Work out the finished part from the listing and answer in its coordinate system (mm). Round coordinates to 2 decimals unless told otherwise and drop trailing zeros. Order: outer loops, then holes, each group sorted by start corner. A loop starts at its lowest first (then second) coordinate and runs counter-clockwise, first axis right, second up. Notation, with made-up numbers: (-14.75, -3.75) - (27.25, -3.75) arc R27 ccw to (27.25, 33.25) - close; hole circle Ø2 at (57, -7.75). An arc over 180 degrees is marked (long way). Put each result on its own line as item: value.
Autodesk Inventor part; units mm, degrees
ref_plane "YZ Plane" through (0, 0, 0) normal (1, 0, 0) x (0, 1, 0)
ref_plane "XZ Plane" through (0, 0, 0) normal (0, 1, 0) x (-1, 0, 0)
ref_plane "XY Plane" through (0, 0, 0) normal (0, 0, 1) x (1, 0, 0)
sketch "Sketch3" plane through (-10.4876, -69.85, 2.286) normal (0, -1, 0) x (1, 0, 0)
  line L0 (0, 0) -> (22.7558, 0)
  line L1 (0, -2.286) -> (0, 0)
  line L2 (0, -2.286) -> (22.7558, -2.286)
  line L3 (22.7558, -2.286) -> (22.7558, 0)
  line L4 (22.7558, 0) -> (23.3146, 0)
  line L5 (22.7558, -2.286) -> (22.7558, 0)
  line L6 (22.7558, -2.286) -> (23.3146, -2.286)
  line L7 (23.3146, -2.286) -> (23.3146, 0)
  line L8 (0, 0) -> (-2.0854, 0)
  line L9 (-2.0854, -2.286) -> (-2.0854, 0)
  line L10 (0, -2.286) -> (-2.0854, -2.286)
  line L11 (0, -2.286) -> (0, 0)
  point P0 (10.4876, -2.286)
extrude "Extrusion3" add sketch "Sketch3" along normal mid plane 38.1
sketch "Sketch4" plane through (65.7357, -25.8425, 2.286) normal (0.866, -0.5, 0) x (0, 0, -1)
  line L0 (2.286, 0) -> (0, 0)
  line L1 (0, -22.7558) -> (0, 0)
  line L2 (2.286, -22.7558) -> (0, -22.7558)
  line L3 (2.286, -22.7558) -> (2.286, 0)
  line L4 (0, 0) -> (0, 2.0854)
  line L5 (2.286, 0) -> (0, 0)
  line L6 (2.286, 0) -> (2.286, 2.0854)
  line L7 (2.286, 2.0854) -> (0, 2.0854)
  line L8 (0, -23.3146) -> (0, -22.7558)
  line L9 (2.286, -23.3146) -> (0, -23.3146)
  line L10 (2.286, -23.3146) -> (2.286, -22.7558)
  line L11 (2.286, -22.7558) -> (0, -22.7558)
  point P0 (2.286, -10.4876)
extrude "Extrusion4" add sketch "Sketch4" along normal mid plane 38.1
sketch "Sketch5" plane through (12.827, -88.9, 0) normal (0, 0, -1) x (-1, 0, 0)
  arc A0 (-30.132, 61.7072) -> (-32.2021, 65.2928) centre (-31.1671, 63.5) ccw
  line L0 (-32.2021, 65.2928) -> (-30.132, 61.7072)
  line L1 (7.3756, 100.2707) -> (-70.4492, 55.3385)
  line L2 (-57.7492, 33.3415) -> (-70.4492, 55.3385)
  line L3 (-4.7625, 63.9334) -> (-57.7492, 33.3415)
  arc A1 (0, 61.1837) -> (-4.7625, 63.9334) centre (-3.175, 61.1837) ccw
  line L4 (0, 61.1837) -> (0, 0)
  line L5 (25.4, 0) -> (0, 0)
  line L6 (25.4, 89.8643) -> (25.4, 0)
  line L7 (24.8412, 91.9497) -> (25.4, 89.8643)
  line L8 (9.461, 100.8295) -> (24.8412, 91.9497)
  line L9 (9.461, 100.8295) -> (7.3756, 100.2707)
  arc A2 (14.8971, 38.1) -> (10.7569, 38.1) centre (12.827, 38.1) ccw
  line L10 (10.7569, 38.1) -> (14.8971, 38.1)
  circle A3 centre (-9.17, 76.2) radius 2.0701
  circle A4 centre (12.827, 88.9) radius 2.0701
  circle A5 centre (12.827, 63.5) radius 2.0701
extrude "Extrusion5" add sketch "Sketch5" against normal blind 2.286
sketch "Sketch6" plane through (12.827, -88.9, 0) normal (0, 0, -1) x (-1, 0, 0)
  arc A0 (-30.132, 61.7072) -> (-32.2021, 65.2928) centre (-31.1671, 63.5) ccw
  line L0 (-57.7492, 33.3415) -> (-70.4492, 55.3385)
  line L1 (-4.7625, 63.9334) -> (-57.7492, 33.3415)
  line L2 (25.4, 89.8643) -> (25.4, 0)
  arc A1 (14.8971, 38.1) -> (10.7569, 38.1) centre (12.827, 38.1) ccw
  circle A2 centre (-9.17, 76.2) radius 2.0701
  circle A3 centre (12.827, 88.9) radius 2.0701
  circle A4 centre (12.827, 63.5) radius 2.0701
  circle A5 centre (12.827, 88.9) radius 2.54
  circle A6 centre (-9.17, 76.2) radius 2.54
  circle A7 centre (12.827, 63.5) radius 2.54
  circle A8 centre (12.827, 38.1) radius 2.54
  circle A9 centre (-31.1671, 63.5) radius 2.54
  circle A10 centre (-53.1006, 50.69) radius 2.54
  circle A11 centre (12.7, 12.7) radius 2.54
  dimension "d20" = 5.08
  dimension "d21" = 5.08
  dimension "d22" = 5.08
  dimension "d23" = 5.08
  dimension "d24" = 5.08
  dimension "d25" = 5.08
  dimension "d26" = 5.08
  dimension "d27" = 12.7
  dimension "d28" = 25.4
  dimension "d29" = 12.7
  dimension "d30" = 12.7
extrude "Extrusion6" cut sketch "Sketch6" against normal blind 2.286 contours A2 | A3 | A4 | A5 | A6 | A7 | A8 | A9 | A10 | A11
sketch "Sketch7" plane through (12.827, -88.9, 0) normal (0, 0, -1) x (-1, 0, 0)
  circle A0 centre (12.827, 38.1) radius 2.54
  circle A1 centre (-31.1671, 63.5) radius 2.54
  line L0 (-4.7625, 63.9334) -> (-57.7492, 33.3415)
  arc A2 (0, 61.1837) -> (-4.7625, 63.9334) centre (-3.175, 61.1837) ccw
  line L1 (0, 61.1837) -> (0, 0)
  line L2 (-31.1671, 63.5) -> (12.827, 38.1) construction
  line L3 (-18.3401, 56.0943) -> (0, 66.683)
  line L4 (0, 66.683) -> (0, 45.5057)
  line L5 (0, 61.1837) -> (0, 0)
  line L6 (0, 45.5057) -> (-18.3401, 56.0943)
extrude "Extrusion7" add sketch "Sketch7" against normal blind 2.286 contours A2 L1 L6 L0
properties part number "Versaframe 60deg gusset" material "Aluminum 6061"
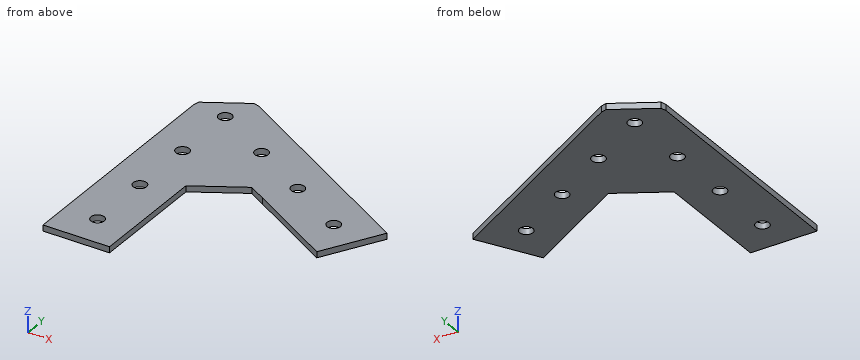
1) A cutting plane is placed at B-B on x = 0. Write down the section's boundary in (y, z), then the cut area to 3 significant figures.
Findings below:
outline: (-88.9, 0) - (-78.74, 0) - (-78.74, 2.29) - (-88.9, 2.29) - close; (-73.66, 0) - (-53.34, 0) - (-53.34, 2.29) - (-73.66, 2.29) - close; (-48.26, 0) - (-27.94, 0) - (-27.94, 2.29) - (-48.26, 2.29) - close; (-22.86, 0) - (-2.54, 0) - (-2.54, 2.29) - (-22.86, 2.29) - close; (2.54, 0) - (9.99, 0) - (9.99, 2.29) - (2.54, 2.29) - close
area: 180 mm2
2) Straight lines are drawn through the part: L1, parallel to Y at x = 0, z = 1.25; L2, parallel to X at y = -52, z = 0.95; L3, parallel to Y at x = 42.5, z = 0.6. For each, find the intervals that lie inside material, in ascending order. Write a range as from..to.
Findings below:
L1: y = -88.9..-78.74, -73.66..-53.34, -48.26..-27.94, -22.86..-2.54, 2.54..9.99
L2: x = -12.57..-2.24, 2.24..12.83, 64.41..72.63
L3: y = -39.35..-27.45, -23.35..-10.02
3) A cutting plane is placed at D-D on y = -12.7. Write down the section's boundary in (x, z).
Findings below:
outline: (-12.57, 0) - (19.46, 0) - (19.46, 2.29) - (-12.57, 2.29) - close; (24.54, 0) - (47.14, 0) - (47.14, 2.29) - (24.54, 2.29) - close
4) A cutting plane is placed at A-A on y = -25.4. Write down the section's boundary in (x, z).
Findings below:
outline: (-12.57, 0) - (-2.54, 0) - (-2.54, 2.29) - (-12.57, 2.29) - close; (2.54, 0) - (41.45, 0) - (41.45, 2.29) - (2.54, 2.29) - close; (46.53, 0) - (69.14, 0) - (69.14, 2.29) - (46.53, 2.29) - close
5) A cutting plane is placed at C-C on z = 1.25. Give the number of separate pieces and of enclosed holes in the cut face, then the cut area to 3 significant figures.
Findings below:
separate pieces: 1
enclosed holes: 7
area: 4,400 mm2
6) Given pin 1 Ø4 at (x, y) = (43.99, -25.4) entering from -Z; pin 2 Ø0.7 at (y, z) = (-55.5, 0.5) entering from +X, each flat-ended and moving along its own axis, determine where each tip first touches the part or whether it passes through.
Findings below:
pin 1: passes through
pin 2: stops at x = 70.81
